Here's the drawing with two shaded views (mm, measured from the low corner). I have some questions. A direction names the side the tool comes from. Give positions to 0.01 mm unless a question says otherwise; leave off trailing zeros. Write each loop counter-clockwise with the first axis right and the second up, starting at its lowest first coordinate (ties: lowest second). Pieces come first, ordered by that corner, then holes.
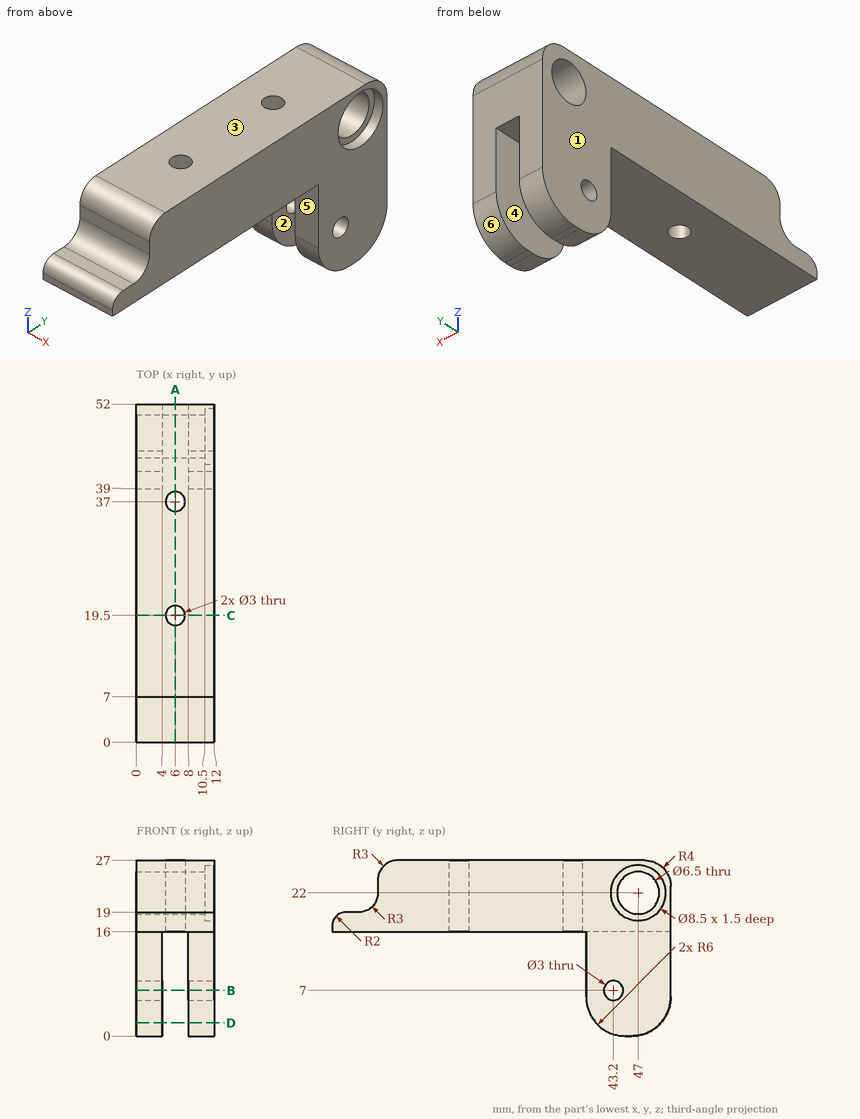
(1) If we mould it in two halves opening along X, with no side actions, what happens to the marked faces 1, 2 and 3? For each: +X half, -X half, draft (parallel to the pull), parting line (faces both ways), or undercut.
Returned:
face 1: -X half
face 2: undercut
face 3: draft
(2) Imagine slicing it at C-C, the plane y = 19.5. Write out the boundary of the cut face in (x, z).
Returned:
outline: (0, 16) - (4.5, 16) - (4.5, 27) - (0, 27) - close; (7.5, 16) - (12, 16) - (12, 27) - (7.5, 27) - close
(3) Imagine slicing it at A-A, the plane x = 6. Write out the boundary of the cut face in (y, z), plus the area to 3 significant figures.
Returned:
outline: (0, 16) - (18, 16) - (18, 27) - (10, 27) arc R3 ccw to (7, 24) - (7, 22) arc R3 cw to (4, 19) - (2, 19) arc R2 ccw to (0, 17) - close; (21, 16) - (35.5, 16) - (35.5, 27) - (21, 27) - close; (38.5, 16) - (52, 16) - (52, 23) arc R4 ccw to (48, 27) - (38.5, 27) - close; hole circle Ø6.5 at (47, 22)
area: 413 mm2
(4) For the marked faces 4, 5 and 6, which set-ups out of +Z, -Z, +X, -X, +Y, -Y let a thin tool reach every point of the face, with its end or its side?
Returned:
face 4: -Z, +Y, -Y
face 5: -Z, +X, -X, -Y
face 6: -Z, +X, -X, +Y
(5) Will these pins go through, and if not, where does the flat tip stop? P1, Ø2, axis at x = 2, z = 12, coming from the -Y side; P2, Ø2.5, axis at x = 6, y = 37, coming from the +Z side; P3, Ø2, axis at x = 6, z = 23, coming from the -Y side; P4, Ø5, axis at x = 6, y = 19.5, coming from the -Z side.
Returned:
P1: stops at y = 39
P2: passes through
P3: stops at y = 7
P4: stops at z = 16
(6) Imagine slicing it at D-D, the plane z = 2. Write out the boundary of the cut face in (x, y).
Returned:
outline: (0, 40.53) - (4, 40.53) - (4, 50.47) - (0, 50.47) - close; (8, 40.53) - (12, 40.53) - (12, 50.47) - (8, 50.47) - close
(7) Imagine slicing it at B-B, the plane z = 7. Write out the boundary of the cut face in (x, y), plus the area to 3 significant figures.
Returned:
outline: (0, 39) - (4, 39) - (4, 41.7) - (0, 41.7) - close; (0, 44.7) - (4, 44.7) - (4, 52) - (0, 52) - close; (8, 39) - (12, 39) - (12, 41.7) - (8, 41.7) - close; (8, 44.7) - (12, 44.7) - (12, 52) - (8, 52) - close
area: 80.0 mm2
(8) If I drill on L1, parallel to X at y = 45, z = 4.5; L2, parallel to Z at x = 4.25, y = 47; L3, parallel to Z at x = 4.25, y = 23.5, over which ranges is the centre line in solid material (lowest first)?
Returned:
L1: x = 0 to 4, 8 to 12
L2: z = 16 to 18.75, 25.25 to 27
L3: z = 16 to 27
